from build123d import *

# Parameters (mm, degrees)
BOSS_EXTRUDE1_DEPTH      = 2.6
BOSS_EXTRUDE1_DEPTH_BACK = 6
FILLET1_R                = 20
CUT_EXTRUDE1_DEPTH       = 5
SKETCH5_R                = 2
CUT_EXTRUDE2_DEPTH       = 20
FILLET3_R                = 1
CIRPATTERN1_COUNT        = 3
SKETCH6_R                = 2.75
CUT_EXTRUDE3_DEPTH       = 56.475677209
BOSS_EXTRUDE2_DEPTH      = 4
SKETCH8_R                = 2.1
CUT_EXTRUDE4_DEPTH       = 70.075616261
CHAMFER1_SIZE            = 2.5
SKETCH9_R                = 1.5
CUT_EXTRUDE5_DEPTH       = 70.075616261


with BuildPart() as part:
    # Sketch3 → Boss-Extrude1 (new, two sides: drawn at the far end of the back side and taken through both)
    with BuildSketch(Plane.XY.offset(-BOSS_EXTRUDE1_DEPTH_BACK)):
        Polygon((-25, 39), (25, 39), (25, -3.511595657), (38.504425224, -11.308379196), (33.774990748, -19.5), (29.045556271, -27.691620804), (-29.045556271, -27.691620804), (-33.774990748, -19.5), (-38.504425224, -11.308379196), (-25, -3.511595657), align=None)
    extrude(amount=BOSS_EXTRUDE1_DEPTH + BOSS_EXTRUDE1_DEPTH_BACK)

    # Fillet1
    fillet1_edges = [part.edges().sort_by_distance(p)[0] for p in [
        (25, -3.511595657, -1.7),
        (-25, -3.511595657, -1.7),
    ]]
    fillet(fillet1_edges, radius=FILLET1_R)

    # Sketch4 → Cut-Extrude1 (cut, symmetric)
    with BuildSketch(Plane(origin=(0, 30, 0), x_dir=(1, 0, 0), z_dir=(0, 1, 0))):
        Polygon((5.114783638, 0.485216362), (-5.114783638, 0.485216362), (-6, -0.4), (-6, -2.6), (6, -2.6), (6, -0.4), align=None)
    cut_extrude1 = extrude(amount=CUT_EXTRUDE1_DEPTH, both=True, mode=Mode.SUBTRACT)

    # Sketch5 → Cut-Extrude2 (cut)
    with BuildSketch(Plane(origin=(0, 39, 0), x_dir=(1, 0, 0), z_dir=(0, 1, 0))):
        with Locations(Location((-4.458868953, 0, 0), (0, 0, 180))):
            Circle(SKETCH5_R)
        with Locations(Location((4.458868953, 0, 0), (0, 0, 180))):
            Circle(SKETCH5_R)
    cut_extrude2 = extrude(amount=-CUT_EXTRUDE2_DEPTH, mode=Mode.SUBTRACT)

    # Fillet3
    fillet3_edges = [part.edges().sort_by_distance(p)[0] for p in [
        (-6, 30, 2.6),
        (6, 30, 2.6),
    ]]
    fillet(fillet3_edges, radius=FILLET3_R)

    # CirPattern1: Cut-Extrude1, Cut-Extrude2 ×3 about axis
    cirpattern1_axis = Axis((0, 0, 0), (0, 0, 1))
    add([cut_extrude1.rotate(cirpattern1_axis, i * 360 / CIRPATTERN1_COUNT) for i in range(1, CIRPATTERN1_COUNT)], mode=Mode.SUBTRACT)
    add([cut_extrude2.rotate(cirpattern1_axis, i * 360 / CIRPATTERN1_COUNT) for i in range(1, CIRPATTERN1_COUNT)], mode=Mode.SUBTRACT)

    # Sketch6 → Cut-Extrude3 (cut, through all)
    with BuildSketch(Plane.XY.offset(2.6)):
        Circle(SKETCH6_R)
    extrude(amount=-CUT_EXTRUDE3_DEPTH, mode=Mode.SUBTRACT)

    # Sketch7 → Boss-Extrude2 (add)
    with BuildSketch(Plane(origin=(0, 0, -6), x_dir=(-1, 0, 0), z_dir=(0, 0, -1))):
        with BuildLine():
            Line((-25, 39), (-3.663721376, 55.451541401))
            ThreePointArc((-3.663721376, 55.451541401), (0, 56.7), (3.663721376, 55.451541401))
            Line((3.663721376, 55.451541401), (25, 39))
            Line((25, 39), (-25, 39))
        make_face()
    extrude(amount=-BOSS_EXTRUDE2_DEPTH)

    # Sketch8 → Cut-Extrude4 (cut, through all)
    with BuildSketch(Plane.XY.offset(2.6)):
        with Locations((-19, 5.7)):
            Circle(SKETCH8_R)
        with Locations((19, 5.7)):
            Circle(SKETCH8_R)
        with Locations((0, 50.7)):
            Circle(SKETCH8_R)
    extrude(amount=-CUT_EXTRUDE4_DEPTH, mode=Mode.SUBTRACT)

    # Chamfer1
    chamfer1_edges = [part.edges().sort_by_distance(p)[0] for p in [
        (-21.1, 5.7, 2.6),
        (16.9, 5.7, 2.6),
        (-2.1, 50.7, -2),
    ]]
    chamfer(chamfer1_edges, length=CHAMFER1_SIZE)

    # Sketch9 → Cut-Extrude5 (cut, through all)
    with BuildSketch(Plane(origin=(0, 0, -6), x_dir=(-1, 0, 0), z_dir=(0, 0, -1))):
        with Locations((7.5, -21.041620804)):
            Circle(SKETCH9_R)
        with Locations((-2, -21.041620804)):
            Circle(SKETCH9_R)
    extrude(amount=-CUT_EXTRUDE5_DEPTH, mode=Mode.SUBTRACT)


solid = part.part
For this review, take the finished solid that the model builds, in its own axes (mm). A direction names the side the tool comes from. Round coordinates to 2 decimals unless told otherwise and drop trailing zeros. Loops run counter-clockwise (first coordinate to the right, second up) from the corner with the lowest first, then second, coordinate; pieces in that order, holes last. Notation, with made-up numbers: (-10.5, 3.25) - (-0.5, 3.25) arc R32 cw to (-0.5, 40.25) - close; hole circle Ø9 at (36, -19.5). An arc over 180 degrees is marked (long way). Put each result on its own line as item: value. Start each with the question number.
1. For faces 1 (the flat face through (-14.183, 47.341, -4.028)), 2 (the flat face through (0, 39, 0)), 3 (the flat face through (-29.04, -9.84, 1.95)), list the 3-axis set-ups (+Z, -Z, +X, -X, +Y, -Y) from which the entire face can be reached by the end or side of a thin tool; tool diameter is ignored.
2. Insertion check: P1, Ø5, axis at x = 11, z = 0, coming from the +Y side; P2, Ø2, axis at x = -17.5, z = -4.5, coming from the +Y side; P3, Ø2.5, axis at x = 19, y = 5.7, coming from the -Z side; P4, Ø4.5, axis at x = -4, z = 0.5, coming from the +Y side. Each pin has a flat end and moves straight along its axis. Give the tip position at first contact, or say it passes through.
3. Mouldability with a two-part tool opening along Y and no side actions: class faces 4 (the flat face through (-36.777, -10.311, -1.76)), 5 (the flat face through (-26, -15, -0.485)), 6 (the flat face through (0, -27.692, -2)), 7 (the flat face through (14.21, -13.39, 0.03)) as +Y half, -Y half, draft (parallel to the pull), parting line (faces both ways), or undercut.
4. Consider section C-C on y = 50.7. State the section outline as (x, z) points.
5. Consider section D-D on x = -12. State the section outline as (y, z) points.
6. Consider section A-A on y = 5.7. State the section outline as (x, z) points.
7. Consider section B-B on y = 31.5. State the section outline as (x, z) points.
8. For probe 1 along X at (y, z) = (-20, -3); probe 2 along X at (y, z) = (4, -0.75); probe 3 along X at (y, z) = (30.5, 0), list the stretches that pass through material, from the lowest coordinate up. Write a range as [from, to].
Result sheet:
1. face 1: +Z, -Z, -X, +Y
1. face 2: +Z, +X, -X, +Y
1. face 3: +Z
2. P1: y = 50.95
2. P2: y = 45.55
2. P3: through
2. P4: y = 39
3. face 4: +Y half
3. face 5: undercut
3. face 6: -Y half
3. face 7: undercut
4. outline: (-9.83, -6) - (-2.1, -6) - (-2.1, -4.5) - (-4.6, -2) - (-9.83, -2) - close; (2.1, -6) - (9.83, -6) - (9.83, -2) - (4.6, -2) - (2.1, -4.5) - close
5. outline: (-27.69, -6) - (49.02, -6) - (49.02, -2) - (39, -2) - (39, 2.6) - (-27.69, 2.6) - close
6. outline: (-25.14, -6) - (-21.1, -6) - (-21.1, 0.1) - (-23.6, 2.6) - (-25.14, 2.6) - close; (-16.9, -6) - (16.9, -6) - (16.9, 0.1) - (14.4, 2.6) - (-14.4, 2.6) - (-16.9, 0.1) - close; (21.1, -6) - (25.14, -6) - (25.14, 2.6) - (23.6, 2.6) - (21.1, 0.1) - close
7. outline: (-25, -6) - (25, -6) - (25, 2.6) - (7, 2.6) arc R1 ccw to (6, 1.6) - (6, 1.27) arc R2 cw (long way) to (2.52, -0.49) - (-2.52, -0.49) arc R2 cw (long way) to (-6, 1.27) - (-6, 1.6) arc R1 ccw to (-7, 2.6) - (-25, 2.6) - close
8. probe 1: [-33.49, -8.58], [-6.42, 0.92], [3.08, 33.49]
8. probe 2: [-25.41, -20.23], [-17.77, 17.77], [20.23, 25.41]
8. probe 3: [-25, -6.46], [6.46, 25]
